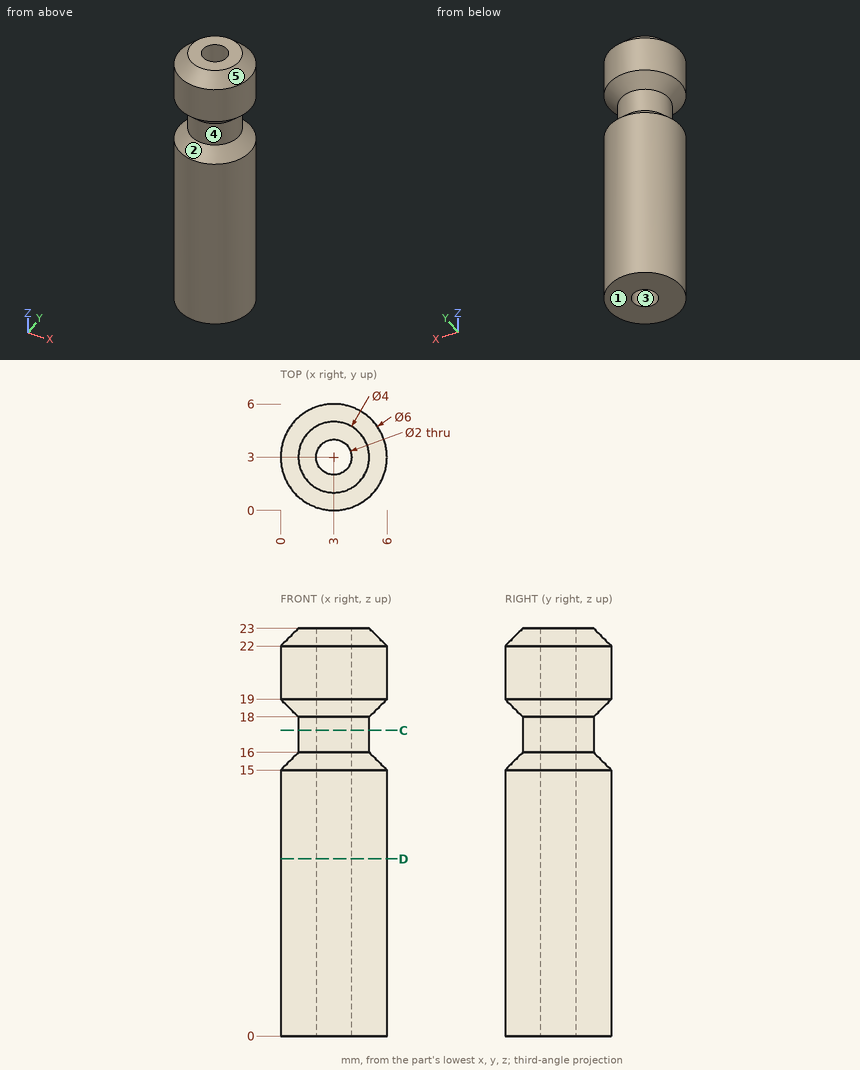
Job drawing, mm, ordinate dimensions from the low corner. One solid piece. A direction names the side the tool comes from. Round coordinates to 2 decimals unless told otherwise and drop trailing zeros. Write each loop counter-clockwise with the first axis right and the second up, starting at its lowest first coordinate (ties: lowest second). Pieces come first, ordered by that corner, then holes. Notation, with made-up numbers: (35.25, 32.5) -> (67.25, 32.5) arc R16 ccw to (67.25, 37.5) -> close; hole circle Ø3 at (43, 67). An arc over 180 degrees is marked (long way). Answer as CSV lines item,"result".
1. Tool access for the marked faces 4 and 5: list every direction of +Z, -Z, +X, -X, +Y, -Y with a clear straight run to the whole face (end or side of a thin tool).
Resolved:
face 4,"none"
face 5,"+Z"
2. Drill centre lines: line 1 (X direction, y = 3.1, z = 7.25) (3 decimals); line 2 (Y direction, x = 3, z = 10); line 3 (Z direction, x = 3.9, y = 5.4). Where is each one in solid material? Low to high.
Resolved:
line 1,"0.002 to 2.005, 3.995 to 5.998"
line 2,"0 to 2, 4 to 6"
line 3,"0 to 15.44, 18.56 to 22.44"
3. Slice it at D-D, the plane z = 10. List the corners of the cut face in (x, y), plus the area to 3 significant figures.
Resolved:
outline,"circle Ø6 at (3, 3); hole circle Ø2 at (3, 3)"
area,"25.1 mm²"
4. Mould opens along Y. For the marked faces 1, 2 and 3 say: +Y half, -Y half, draft (parallel to the pull), parting line (faces both ways), or undercut.
Resolved:
face 1,"draft"
face 2,"parting line"
face 3,"undercut"
5. Pin check, flat tips, straight feed: pin 1 Ø1.5 at (x, z) = (1, 8) entering from +Y; pin 2 Ø1.5 at (y, z) = (2, 20.5) entering from -X; pin 3 Ø1.2 at (x, y) = (3, 3) entering from -Z; pin 4 Ø1.5 at (y, z) = (1, 13.5) entering from +X. Stop position of each tip, or through.
Resolved:
pin 1,"y = 5.73"
pin 2,"x = 0.01"
pin 3,"through"
pin 4,"x = 5.73"
6. Slice it at C-C, the plane z = 17.25. List the corners of the cut face in (x, y).
Resolved:
outline,"circle Ø4 at (3, 3); hole circle Ø2 at (3, 3)"
